The drawing under review shows one solid part. Ordinate dimensions are in mm from its lowest x, y, z. A direction names the side the tool comes from. Give positions to 0.01 mm unless a question says otherwise; leave off trailing zeros. Order: outer loops, then holes, each group sorted by start corner. A loop starts at its lowest first (then second) coordinate and runs counter-clockwise, first axis right, second up. Notation, with made-up numbers: (75.5, 15.5) -> (121.5, 15.5) arc R15 cw to (121.5, 31.5) -> close; hole circle Ø9 at (37, -9.75). An arc over 180 degrees is marked (long way). One line per item, written item: value. Start each with the question number.
1) For pin 1 (1 mm diameter, centred on x = 10, y = 0.5, fed in from -Z), flat-tipped, find the tip position at first contact; note if it passes through.
2) Consider section D-D (y = 2.6). State the section outline as (x, z) points.
3) Wall thickness on line 1 along Z through (x, y) = (7.5, 1.75); line 2 along Y through (x, z) = (8.75, 14); line 3 along Z through (x, y) = (7.5, 2.7): over which ranges is each line inside the solid? List them lowest first. Write a range as from..to.
4) Consider section B-B (x = 7.5). State the section outline as (y, z) points, plus the area to 3 significant figures.
5) Tool access review of the marked faces 4 and 5: name each direction out of +Z, -Z, +X, -X, +Y, -Y from which nothing blocks a thin tool from reaching the whole face with its end or side.
6) Consider section A-A (z = 7.5). State the section outline as (x, y) points.
7) The part is to be moulded in two halves that separate along Z. For the marked faces 1, 2 and 3, say which applies: released by +Z, released by -Z, zero draft, split by the parting line, or undercut.
8) Consider section C-C (y = 0.5). State the section outline as (x, z) points.
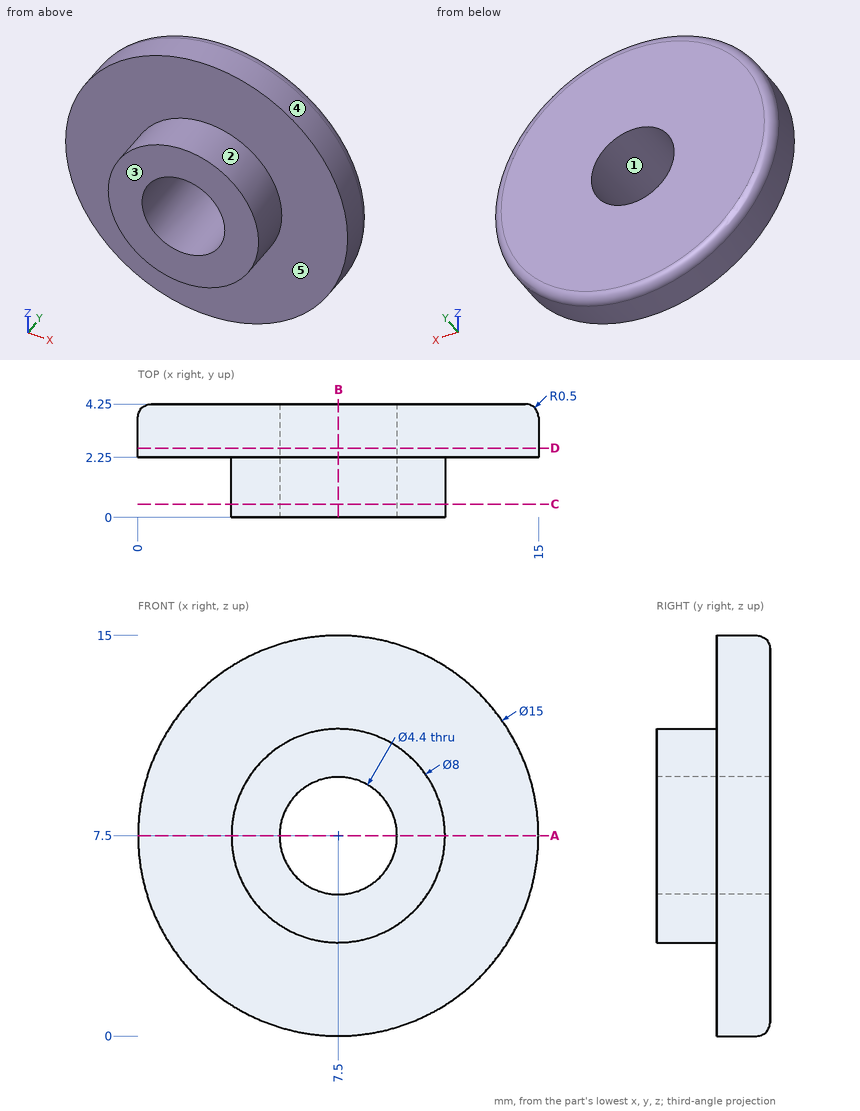
Checked values:
1. pin 1: stops at z = 4.04
2. outline: circle Ø15 at (7.5, 7.5); hole circle Ø4.4 at (7.5, 7.5)
3. line 1: z = 3.5..5.3, 9.7..11.5
3. line 2: y = 2.25..4.25
3. line 3: z = 0..5.3, 9.7..15
4. outline: (0, 3.5) -> (2.25, 3.5) -> (2.25, 0) -> (3.75, 0) arc R0.5 ccw to (4.25, 0.5) -> (4.25, 5.3) -> (0, 5.3) -> close; (0, 9.7) -> (4.25, 9.7) -> (4.25, 14.5) arc R0.5 ccw to (3.75, 15) -> (2.25, 15) -> (2.25, 11.5) -> (0, 11.5) -> close
4. area: 29.2 mm^2
5. face 4: +Y, -Y
5. face 5: -Y
6. outline: (0, 2.25) -> (3.5, 2.25) -> (3.5, 0) -> (5.3, 0) -> (5.3, 4.25) -> (0.5, 4.25) arc R0.5 ccw to (0, 3.75) -> close; (9.7, 0) -> (11.5, 0) -> (11.5, 2.25) -> (15, 2.25) -> (15, 3.75) arc R0.5 ccw to (14.5, 4.25) -> (9.7, 4.25) -> close
7. face 1: undercut
7. face 2: split by the parting line
7. face 3: zero draft
8. outline: circle Ø8 at (7.5, 7.5); hole circle Ø4.4 at (7.5, 7.5)
